Can you work these out from the model? Positions are in its coordinate system, mm. A direction names the side the tool comes from. Give positions to 0.01 mm unless a question says otherwise; leave off trailing zeros. Loops run counter-clockwise (first coordinate to the right, second up) from the corner with the lowest first, then second, coordinate; pieces in that order, holes last. Notation, with made-up numbers: M 88.25,64 L 110.25,64 A15 cw 110.25,85 Z; hole C -33,7.25 d9. An arc over 180 degrees is marked long. Put each result on its own line as item: value. Start each with the question number.
1) For faces 1 (the cylindrical face through (-4.255, -12.694, 1.972)), 2 (the cylindrical face through (-2.68, -13.15, 1.97)), 3 (the cylindrical face through (10.05, -8.9, 1.97)), 4 (the cylindrical face through (-11.986, 1.586, 1.972)), which set-ups out of +Z, -Z, +X, -X, +Y, -Y let a thin tool reach every point of the face, with its end or its side?
2) Please list where these lines run through material, in increasing order: line 1 along Y through (x, z) = (30.75, 1.45); line 2 along X through (y, z) = (-12.5, 2.1); line 3 along X through (y, z) = (-13.5, 1.9). Write a range as from..to.
3) If we mould it in two halves opening along X, with no side actions, what happens to faces 5 (the cylindrical face through (-0.825, -13.363, 1.972)), 6 (the cylindrical face through (-10.032, -8.866, 1.972)), 7 (the flat face through (23, 4, 2))? For each: +X half, -X half, draft (parallel to the pull), parting line (faces both ways), or undercut.
4) Imagine slicing it at B-B (x = 15). Write out the boundary of the cut face in (y, z), then the cut area to 3 significant figures.
5) Imagine slicing it at A-A (z = 1.6). State how many separate pieces and enclosed holes the cut face has, then the cut area to 3 significant figures.
6) For P1, Ø2, axis at y = -11.5, z = 2, coming from the +X side; P2, Ø4.5, axis at x = 30.75, y = 0, coming from the +Z side; P3, Ø2, axis at x = 23, z = 1.5, coming from the +Y side; P4, Ø1.2, axis at x = 23, z = 3, coming from the -Y side, each with a flat end and sliding along its axis, tell me the tip position at first contact or that it passes through.
from build123d import *

# Parameters (mm, degrees)
SKETCH1_R           = 1.75
BOSS_EXTRUDE1_DEPTH = 4
SKETCH6_R           = 1.3
SKETCH6_R_2         = 2.4
CUT_EXTRUDE1_DEPTH  = 38.915688046


with BuildPart() as part:
    # Sketch1 → Boss-Extrude1 (new body)
    with BuildSketch(Plane.XY):
        with BuildLine():
            ThreePointArc((14.048088143, -4.085109489), (14.06038767, -4.04257326), (14.072558403, -4))
            Line((14.072558403, -4), (30.75, -4))
            ThreePointArc((30.75, -4), (34.75, 0), (30.75, 4))
            Line((30.75, 4), (14.072558403, 4))
            ThreePointArc((14.072558403, 4), (14.06038767, 4.04257326), (14.048088143, 4.085109489))
            ThreePointArc((14.048088143, 4.085109489), (12.712915648, 4.255390909), (11.377106712, 4.090176385))
            ThreePointArc((11.377106712, 4.090176385), (0, 12.09), (-11.377106712, 4.090176385))
            ThreePointArc((-11.377106712, 4.090176385), (-12.712915648, 4.255390909), (-14.048088143, 4.085109489))
            ThreePointArc((-14.048088143, 4.085109489), (-14.131494839, 3.78652263), (-14.208555951, 3.486235477))
            ThreePointArc((-14.208555951, 3.486235477), (-13.137403362, 2.671181194), (-11.897951627, 2.1463567))
            ThreePointArc((-11.897951627, 2.1463567), (-11.986568374, 1.578061664), (-12.048056748, 1.00619511))
            ThreePointArc((-12.048056748, 1.00619511), (-13.381109763, 0.820047291), (-14.626715284, 0.31))
            ThreePointArc((-14.626715284, 0.31), (-14.63, 0), (-14.626715284, -0.31))
            ThreePointArc((-14.626715284, -0.31), (-13.381109763, -0.820047291), (-12.048056748, -1.00619511))
            ThreePointArc((-12.048056748, -1.00619511), (-11.986568374, -1.578061664), (-11.897951627, -2.1463567))
            ThreePointArc((-11.897951627, -2.1463567), (-13.137403362, -2.671181194), (-14.208555951, -3.486235477))
            ThreePointArc((-14.208555951, -3.486235477), (-14.131494839, -3.78652263), (-14.048088143, -4.085109489))
            ThreePointArc((-14.048088143, -4.085109489), (-12.712915648, -4.255390909), (-11.377106712, -4.090176385))
            ThreePointArc((-11.377106712, -4.090176385), (-11.169703548, -4.626642697), (-10.937020765, -5.152637848))
            ThreePointArc((-10.937020765, -5.152637848), (-11.998404632, -5.980373095), (-12.82210701, -7.044889767))
            ThreePointArc((-12.82210701, -7.044889767), (-12.669951657, -7.315), (-12.51210701, -7.581825517))
            ThreePointArc((-12.51210701, -7.581825517), (-11.17835734, -7.400736668), (-9.930825655, -6.8954189))
            ThreePointArc((-9.930825655, -6.8954189), (-9.591641884, -7.359925677), (-9.230750012, -7.807775241))
            ThreePointArc((-9.230750012, -7.807775241), (-10.041734454, -8.882012453), (-10.561852666, -10.123446462))
            ThreePointArc((-10.561852666, -10.123446462), (-10.344972209, -10.344972209), (-10.123446462, -10.561852666))
            ThreePointArc((-10.123446462, -10.561852666), (-8.882012453, -10.041734454), (-7.807775241, -9.230750012))
            ThreePointArc((-7.807775241, -9.230750012), (-7.359925677, -9.591641884), (-6.8954189, -9.930825655))
            ThreePointArc((-6.8954189, -9.930825655), (-7.400736668, -11.17835734), (-7.581825517, -12.51210701))
            ThreePointArc((-7.581825517, -12.51210701), (-7.315, -12.669951657), (-7.044889767, -12.82210701))
            ThreePointArc((-7.044889767, -12.82210701), (-5.980373095, -11.998404632), (-5.152637848, -10.937020765))
            ThreePointArc((-5.152637848, -10.937020765), (-4.626642697, -11.169703548), (-4.090176385, -11.377106712))
            ThreePointArc((-4.090176385, -11.377106712), (-4.255390909, -12.712915648), (-4.085109489, -14.048088143))
            ThreePointArc((-4.085109489, -14.048088143), (-3.78652263, -14.131494839), (-3.486235477, -14.208555951))
            ThreePointArc((-3.486235477, -14.208555951), (-2.671181194, -13.137403362), (-2.1463567, -11.897951627))
            ThreePointArc((-2.1463567, -11.897951627), (-1.578061664, -11.986568374), (-1.00619511, -12.048056748))
            ThreePointArc((-1.00619511, -12.048056748), (-0.820047291, -13.381109763), (-0.31, -14.626715284))
            ThreePointArc((-0.31, -14.626715284), (0, -14.63), (0.31, -14.626715284))
            ThreePointArc((0.31, -14.626715284), (0.820047291, -13.381109763), (1.00619511, -12.048056748))
            ThreePointArc((1.00619511, -12.048056748), (1.578061664, -11.986568374), (2.1463567, -11.897951627))
            ThreePointArc((2.1463567, -11.897951627), (2.671181194, -13.137403362), (3.486235477, -14.208555951))
            ThreePointArc((3.486235477, -14.208555951), (3.78652263, -14.131494839), (4.085109489, -14.048088143))
            ThreePointArc((4.085109489, -14.048088143), (4.255390909, -12.712915648), (4.090176385, -11.377106712))
            ThreePointArc((4.090176385, -11.377106712), (4.626642697, -11.169703548), (5.152637848, -10.937020765))
            ThreePointArc((5.152637848, -10.937020765), (5.980373095, -11.998404632), (7.044889767, -12.82210701))
            ThreePointArc((7.044889767, -12.82210701), (7.315, -12.669951657), (7.581825517, -12.51210701))
            ThreePointArc((7.581825517, -12.51210701), (7.400736668, -11.17835734), (6.8954189, -9.930825655))
            ThreePointArc((6.8954189, -9.930825655), (7.359925677, -9.591641884), (7.807775241, -9.230750012))
            ThreePointArc((7.807775241, -9.230750012), (8.882012453, -10.041734454), (10.123446462, -10.561852666))
            ThreePointArc((10.123446462, -10.561852666), (10.344972209, -10.344972209), (10.561852666, -10.123446462))
            ThreePointArc((10.561852666, -10.123446462), (10.041734454, -8.882012453), (9.230750012, -7.807775241))
            ThreePointArc((9.230750012, -7.807775241), (9.591641884, -7.359925677), (9.930825655, -6.8954189))
            ThreePointArc((9.930825655, -6.8954189), (11.17835734, -7.400736668), (12.51210701, -7.581825517))
            ThreePointArc((12.51210701, -7.581825517), (12.669951657, -7.315), (12.82210701, -7.044889767))
            ThreePointArc((12.82210701, -7.044889767), (11.998404632, -5.980373095), (10.937020765, -5.152637848))
            ThreePointArc((10.937020765, -5.152637848), (11.169703548, -4.626642697), (11.377106712, -4.090176385))
            ThreePointArc((11.377106712, -4.090176385), (12.712915648, -4.255390909), (14.048088143, -4.085109489))
        make_face()
        Circle(SKETCH1_R, mode=Mode.SUBTRACT)
        with Locations((30.75, 0)):
            Circle(SKETCH1_R, mode=Mode.SUBTRACT)
    extrude(amount=BOSS_EXTRUDE1_DEPTH)

    # Sketch6 → Cut-Extrude1 (cut, through all)
    with BuildSketch(Plane.XY.offset(4)):
        with Locations((4.5, 0)):
            Circle(SKETCH6_R)
        with Locations((-4.5, 0)):
            Circle(SKETCH6_R)
        Circle(SKETCH6_R_2)
    extrude(amount=-CUT_EXTRUDE1_DEPTH, mode=Mode.SUBTRACT)


solid = part.part
Recorded:
1. face 1: +Z, -Z
1. face 2: +Z, -Z, -Y
1. face 3: +Z, -Z, +X
1. face 4: +Z, -Z, -X
2. line 1: -4..-1.75, 1.75..4
2. line 2: -7.58..-6.56, -4.25..-2.36, -0.98..0.98, 2.36..4.25, 6.56..7.58
2. line 3: -4.2..-2.9, -0.79..0.79, 2.9..4.2
3. face 5: undercut
3. face 6: -X half
3. face 7: draft
4. outline: M -4,0 L 4,0 L 4,4 L -4,4 Z
4. area: 32.0 mm²
5. separate pieces: 1
5. enclosed holes: 4
5. area: 645 mm²
6. P1: x = 10.19
6. P2: z = 4
6. P3: y = 4
6. P4: y = -4
